Verification items for the finished model (mm, model axes). Round coordinates to 2 decimals unless told otherwise and drop trailing zeros. Loops run counter-clockwise (first coordinate to the right, second up) from the corner with the lowest first, then second, coordinate; pieces in that order, holes last. Notation, with made-up numbers: M -36,80.5 L -32,80.5 A26 cw -32,97.5 Z; hole C 10,5.5 d2. An arc over 180 degrees is marked long. Answer as CSV lines item,"result".
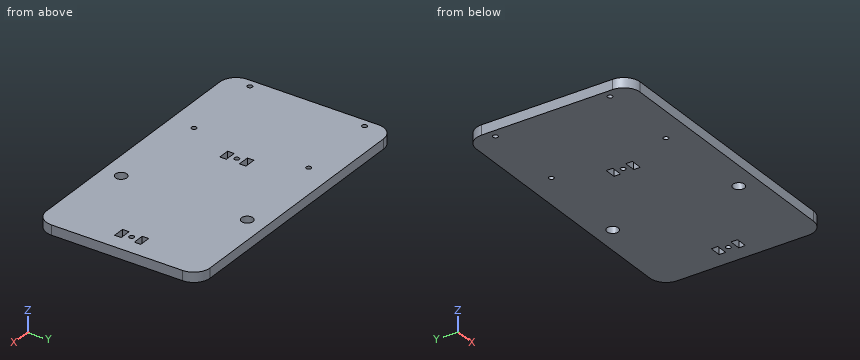
Autodesk Fusion 360 part; units mm, degrees
sketch "Sketch1" plane through (0, 0, 0) normal (0, 0, 1) x (1, 0, 0)
  line L0 (10, 0) -> (165, 0)
  line L1 (175, 10) -> (175, 90)
  line L2 (165, 100) -> (10, 100)
  line L3 (0, 90) -> (0, 10)
  line L4 (5, 85) -> (55, 85)
  line L5 (55, 85) -> (55, 15)
  line L6 (55, 15) -> (5, 15)
  line L7 (5, 15) -> (5, 85)
  line L8 (5, 50) -> (0, 50)
  circle A0 centre (5, 85) radius 1.5
  circle A1 centre (55, 85) radius 1.5
  circle A2 centre (5, 15) radius 1.5
  circle A3 centre (55, 15) radius 1.5
  line L9 (55, 100) -> (55, 0)
  line L10 (65, 100) -> (65, 0)
  line L11 (165, 0) -> (165, 100)
  line L12 (65, 57.5) -> (71, 57.5)
  line L13 (71, 57.5) -> (71, 42.5)
  line L14 (71, 42.5) -> (65, 42.5)
  line L15 (65, 42.5) -> (65, 57.5)
  line L16 (65, 57.5) -> (71, 57.5)
  line L17 (71, 57.5) -> (71, 54.5)
  line L18 (71, 54.5) -> (65, 54.5)
  line L19 (65, 54.5) -> (65, 57.5)
  line L20 (71, 42.5) -> (65, 42.5)
  line L21 (65, 42.5) -> (65, 45.5)
  line L22 (65, 45.5) -> (71, 45.5)
  line L23 (71, 45.5) -> (71, 42.5)
  line L24 (65, 100) -> (165, 100)
  line L25 (115, 100) -> (115, 0)
  line L26 (159, 57.5) -> (159, 42.5)
  line L27 (159, 54.5) -> (165, 54.5)
  line L28 (165, 57.5) -> (159, 57.5)
  line L29 (165, 45.5) -> (159, 45.5)
  line L30 (159, 42.5) -> (165, 42.5)
  circle A4 centre (115, 88.5) radius 3.5
  circle A5 centre (115, 11.5) radius 3.5
  line L31 (115, 88.5) -> (115, 11.5)
  arc A6 (10, 100) -> (0, 90) centre (10, 90) ccw
  arc A7 (0, 10) -> (10, 0) centre (10, 10) ccw
  arc A8 (175, 90) -> (165, 100) centre (165, 90) ccw
  arc A9 (165, 0) -> (175, 10) centre (165, 10) ccw
  line L32 (64.5, 58) -> (71.5, 58)
  line L33 (71.5, 58) -> (71.5, 54)
  line L34 (71.5, 54) -> (64.5, 54)
  line L35 (64.5, 54) -> (64.5, 58)
  line L36 (71.5, 42) -> (64.5, 42)
  line L37 (64.5, 42) -> (64.5, 46)
  line L38 (64.5, 46) -> (71.5, 46)
  line L39 (71.5, 46) -> (71.5, 42)
  line L40 (159, 57.5) -> (165, 57.5)
  line L41 (165, 57.5) -> (165, 54.5)
  line L42 (165, 54.5) -> (159, 54.5)
  line L43 (159, 54.5) -> (159, 57.5)
  line L44 (159, 45.5) -> (165, 45.5)
  line L45 (165, 45.5) -> (165, 42.5)
  line L46 (165, 42.5) -> (159, 42.5)
  line L47 (159, 42.5) -> (159, 45.5)
  line L48 (158.5, 46) -> (165.5, 46)
  line L49 (165.5, 46) -> (165.5, 42)
  line L50 (165.5, 42) -> (158.5, 42)
  line L51 (158.5, 42) -> (158.5, 46)
  line L52 (158.5, 58) -> (165.5, 58)
  line L53 (165.5, 58) -> (165.5, 54)
  line L54 (165.5, 54) -> (158.5, 54)
  line L55 (158.5, 54) -> (158.5, 58)
  point P0 (0, 100)
  point P1 (65, 50)
  point P2 (65, 50)
  point P3 (115, 50)
  point P4 (115, 50)
  dimension "d1" = 50
  dimension "d2" = 70
  dimension "d3" = 100
  dimension "d4" = 90
  dimension "d5" = 5
  dimension "d6" = 3
  dimension "d7" = 3
  dimension "d8" = 3
  dimension "d9" = 3
  dimension "d11" = 120
  dimension "d12" = 10
  dimension "d13" = 10
  dimension "d14" = 6
  dimension "d15" = 15
  dimension "d16" = 3
  dimension "d17" = 3
  dimension "d18" = 77
  dimension "d19" = 7
  dimension "d20" = 7
  dimension "d21" = 10
  dimension "d22" = 10
  dimension "d23" = 10
  dimension "d24" = 10
  dimension "d27" = -0.5
  dimension "d28" = -0.5
  dimension "d29" = -0.5
  dimension "d30" = -0.5
extrude "Extrude1" add sketch "Sketch1" along normal blind 6 contours L0 L3 L6 L7 L8 A2 A3 L9 A7 | L0 L2 L5 A1 A3 L9 L10 L15 L32 L34 L35 L36 L37 L38 | L0 L2 L10 L13 L24 L25 A4 A5 L31 L32 L33 L34 L36 L38 L39 | L2 L3 L4 L7 L8 A0 A1 L9 A6 | L0 L2 L11 L24 L25 L26 A4 A5 L31 L48 L50 L51 L52 L54 L55 | L4 L5 L6 L7 A0 A1 A2 A3 L9 | L1 L11 A8 A9 L48 L49 L50 L52 L53 L54 | L10 L13 L15 L34 L38 | L11 L26 L48 L54
sketch "Sketch2" plane through (0, 0, 6) normal (0, 0, 1) x (-1, 0, 0)
  circle A0 centre (-5, -85) radius 1.5
  line L0 (-64.5, -46) -> (-71.5, -46)
  line L1 (-71.5, -46) -> (-71.5, -42)
  line L2 (-71.5, -42) -> (-64.5, -42)
  line L3 (-64.5, -42) -> (-64.5, -46)
  circle A1 centre (-55, -15) radius 1.5
  circle A2 centre (-5, -15) radius 1.5
  circle A3 centre (-115, -88.5) radius 3.5
  circle A4 centre (-55, -85) radius 1.5
  line L4 (-165.5, -54) -> (-158.5, -54)
  line L5 (-158.5, -54) -> (-158.5, -58)
  line L6 (-158.5, -58) -> (-165.5, -58)
  line L7 (-165.5, -58) -> (-165.5, -54)
  circle A5 centre (-115, -11.5) radius 3.5
  line L8 (-165.5, -42) -> (-158.5, -42)
  line L9 (-158.5, -42) -> (-158.5, -46)
  line L10 (-158.5, -46) -> (-165.5, -46)
  line L11 (-165.5, -46) -> (-165.5, -42)
  line L12 (-71.5, -54) -> (-64.5, -54)
  line L13 (-64.5, -54) -> (-64.5, -58)
  line L14 (-64.5, -58) -> (-71.5, -58)
  line L15 (-71.5, -58) -> (-71.5, -54)
  line L16 (-165, -100) -> (-10, -100)
  arc A6 (-10, -100) -> (0, -90) centre (-10, -90) ccw
  line L17 (0, -90) -> (0, -10)
  arc A7 (0, -10) -> (-10, 0) centre (-10, -10) ccw
  line L18 (-10, 0) -> (-165, 0)
  arc A8 (-165, 0) -> (-175, -10) centre (-165, -10) ccw
  line L19 (-175, -10) -> (-175, -90)
  arc A9 (-175, -90) -> (-165, -100) centre (-165, -90) ccw
  line L20 (-68, -54) -> (-68, -46)
  line L21 (-162, -54) -> (-162, -46)
  circle A10 centre (-162, -50) radius 1.5
  circle A11 centre (-68, -50) radius 1.5
  dimension "d31" = 3
  dimension "d32" = 3
extrude "Extrude2" cut sketch "Sketch2" against normal blind 10 contours L20 A11 | L20 A11 | L21 A10 | L21 A10
equation "d18 = ( ( 70 + 84 ) / 2 ) * 1 mm"
1) Section check A-A (x = 115). Record the cut outline in (y, z), plus the area to 3 significant figures.
Here are the results:
outline,"M 0,0 L 8,0 L 8,6 L 0,6 Z; M 15,0 L 85,0 L 85,6 L 15,6 Z; M 92,0 L 100,0 L 100,6 L 92,6 Z"
area,"516 mm^2"
2) Material ranges on probe 1 along Y at (x, z) = (55, 2.4); probe 2 along Y at (x, z) = (5, 2.65); probe 3 along X at (y, z) = (49.5, 4.55), recorded low to high.
Here are the results:
probe 1,"y = 0 to 13.5, 16.5 to 83.5, 86.5 to 100"
probe 2,"y = 1.34 to 13.5, 16.5 to 83.5, 86.5 to 98.66"
probe 3,"x = 0 to 66.59, 69.41 to 160.59, 163.41 to 175"
3) Section check B-B (z = 2.05). State how many separate pieces and enclosed holes the cut face has, plus the area to 3 significant figures.
Here are the results:
separate pieces,"1"
enclosed holes,"12"
area,"17,200 mm^2"
